CAD build for the part. Positions are in the model's coordinates, mm. Face numbers are marked on the shaded views. A direction names the side the tool comes from. Give positions to 0.01 mm unless a question says otherwise; leave off trailing zeros. Write each loop counter-clockwise with the first axis right and the second up, starting at its lowest first coordinate (ties: lowest second). Pieces come first, ordered by that corner, then holes. Notation, with made-up numbers: (62, 38) - (108, 38) arc R20 cw to (108, 73) - close; hole circle Ø4 at (36.5, -37). An arc over 180 degrees is marked (long way). Answer as a JSON object with one key per item and string values.
from build123d import *

# Parameters (mm, degrees)
SKETCH2_R           = 16
BOSS_EXTRUDE1_DEPTH = 90
SKETCH3_R           = 5
BOSS_EXTRUDE2_DEPTH = 20
BOSS_EXTRUDE4_DEPTH = 10


with BuildPart() as part:
    # Sketch2 → Boss-Extrude1 (new body)
    with BuildSketch(Plane.XY):
        with Locations(Location((0, 0, 0), (0, 0, 180))):
            Circle(SKETCH2_R)
    extrude(amount=BOSS_EXTRUDE1_DEPTH)

    # Sketch3 → Boss-Extrude2 (add)
    with BuildSketch(Plane(origin=(0, 0, 0), x_dir=(-1, 0, 0), z_dir=(0, 0, -1))):
        Circle(SKETCH3_R)
    extrude(amount=BOSS_EXTRUDE2_DEPTH)

    # Sketch5 → Boss-Extrude4 (add)
    with BuildSketch(Plane(origin=(0, 0, -20), x_dir=(-1, 0, 0), z_dir=(0, 0, -1))):
        Polygon((1, 1), (12.7, 1), (12.7, -1), (1, -1), (1, -12.7), (-1, -12.7), (-1, -1), (-12.7, -1), (-12.7, 1), (-1, 1), (-1, 12.7), (1, 12.7), align=None)
    extrude(amount=BOSS_EXTRUDE4_DEPTH)


solid = part.part
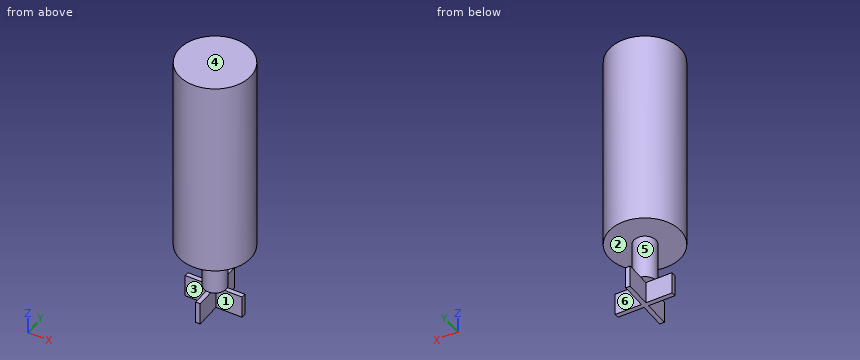
(1) 3-axis set-ups, long thin cutter, end or side, ignore diameter. For the marked faces 1, 2 and 3: which of +Z, -Z, +X, -X, +Y, -Y reach the whole face in a straight line?
Answer key:
{"face 1": "-Z, +X, -Y", "face 2": "none", "face 3": "-Z, -X, -Y"}
(2) Saw through at D-D, the plane z = 79.5. Give the cut face in (x, y).
Answer key:
{"outline": "circle Ø32 at (0, 0)"}
(3) Probe L1, parallel to Z at x = 2.5, y = 15; L2, parallel to Z at x = -4, y = 2; L3, parallel to X at y = -11, z = 74.5. List the from-to ranges inside material, lowest first. Write a range as [from, to].
Answer key:
{"L1": "z = [0, 90]", "L2": "z = [-20, 90]", "L3": "x = [-11.62, 11.62]"}
(4) Saw through at C-C, the plane y = 9. Give the cut face in (x, z).
Answer key:
{"outline": "(-13.23, 0) - (13.23, 0) - (13.23, 90) - (-13.23, 90) - close; (-1, -30) - (1, -30) - (1, -20) - (-1, -20) - close"}
(5) Flat gauge pins, fed straight in: P1, Ø11, axis at y = 7.5, z = -25, coming from the -X side; P2, Ø5, axis at y = -5.5, z = -24.5, coming from the +X side; P3, Ø12, axis at x = -10.5, z = 45.5, coming from the +Y side. Where does each tip first touch, or does it go through?
Answer key:
{"P1": "stops at x = -1", "P2": "stops at x = 1", "P3": "stops at y = 15.35"}
(6) Pull direction Z, two halves, no side cores. Call the marked faces 4, 5 and 6: pulls with the +Z half, pulls with the -Z half, needs draft (parallel to the pull), parting line crosses it, or undercut.
Answer key:
{"face 4": "pulls with the +Z half", "face 5": "undercut", "face 6": "needs draft"}
(7) Saw through at A-A, the plane y = -11. Give the cut face in (x, z).
Answer key:
{"outline": "(-11.62, 0) - (11.62, 0) - (11.62, 90) - (-11.62, 90) - close; (-1, -30) - (1, -30) - (1, -20) - (-1, -20) - close"}
(8) Saw through at B-B, the plane z = -22. Give the cut face in (x, y), and give its area (3 significant figures).
Answer key:
{"outline": "(-12.7, -1) - (-1, -1) - (-1, -12.7) - (1, -12.7) - (1, -1) - (12.7, -1) - (12.7, 1) - (1, 1) - (1, 12.7) - (-1, 12.7) - (-1, 1) - (-12.7, 1) - close", "area": "97.6 mm²"}
